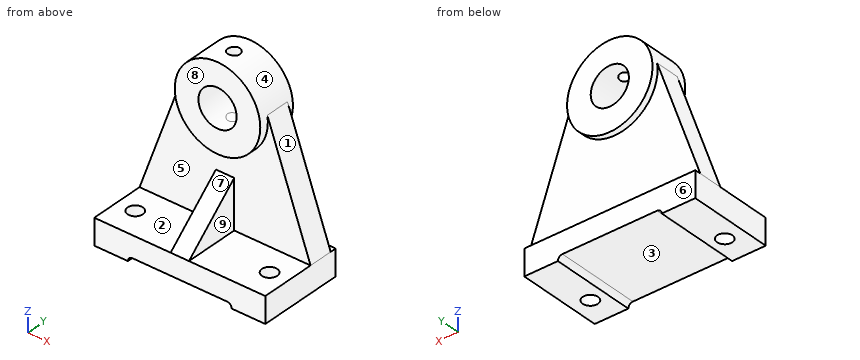
from build123d import *

# Parameters (mm, degrees)
F1_DEPTH  = 28
F3_DEPTH  = 28
F5_DEPTH  = 8
F7_DEPTH  = 4
F8_R      = 28
F9_DEPTH  = 28
F10_R     = 28
F11_DEPTH = 2
F12_R     = 12.5
F13_DEPTH = 26.001
F15_DEPTH = 112
F17_DEPTH = 50
F19_DEPTH = 50
F20_R     = 4
F21_DEPTH = 139
F22_R     = 4
F23_DEPTH = 91
F24_R     = 12.5
F25_DEPTH = 26.0010001
F26_R     = 5
F27_DEPTH = 120.0010001
F28_W     = 68
F28_H     = 3
F29_DEPTH = 28.0010001
F30_R     = 2.99999


# Not quite as in the source:
# - a fillet or chamfer is up to 0.001 mm smaller than in the source, because OpenCascade refuses the exact size


with BuildPart() as f1:
    # F0 (on Front) → F1 (new body, symmetric)
    with BuildSketch(Plane.XZ):
        Polygon((0, 17), (0, 0), (22, 0), (22, 3), (90, 3), (90, 0), (112, 0), (112, 17), align=None)
    extrude(amount=F1_DEPTH, both=True)

    # F2 (on Front) → F3 (join)
    with BuildSketch(Plane.XZ):
        with BuildLine():
            Line((28.3328655167, 96.304610259), (0, 17))
            Line((0, 17), (112, 17))
            Line((112, 17), (83.6671344833, 96.304610259))
            ThreePointArc((83.6671344833, 96.304610259), (56, 64), (28.3328655167, 96.304610259))
        make_face()
    extrude(amount=-F3_DEPTH)

    # F4 (on face) → F5 (cut)
    with BuildSketch(Plane.XZ):
        with BuildLine():
            ThreePointArc((83.6671344833, 96.304610259), (56, 64), (28.3328655167, 96.304610259))
            Line((28.3328655167, 96.304610259), (0, 17))
            Line((0, 17), (112, 17))
            Line((112, 17), (83.6671344833, 96.304610259))
        make_face()
    extrude(amount=-F5_DEPTH, mode=Mode.SUBTRACT)

    # F6 (on face) → F7 (cut)
    with BuildSketch(Plane(origin=(0, 28, 0), x_dir=(-1, 0, 0), z_dir=(0, 1, 0))):
        with BuildLine():
            Line((-83.6671344833, 96.304610259), (-112, 17))
            Line((-112, 17), (0, 17))
            Line((0, 17), (-28.3328655167, 96.304610259))
            ThreePointArc((-28.3328655167, 96.304610259), (-56, 64), (-83.6671344833, 96.304610259))
        make_face()
    extrude(amount=-F7_DEPTH, mode=Mode.SUBTRACT)

    # F8 (on Front) → F9 (join)
    with BuildSketch(Plane.XZ):
        with Locations((56, 92)):
            Circle(F8_R)
    extrude(amount=-F9_DEPTH)

    # F10 (on face) → F11 (cut)
    with BuildSketch(Plane.XZ):
        with Locations((56, 92)):
            Circle(F10_R)
    extrude(amount=-F11_DEPTH, mode=Mode.SUBTRACT)

    # F12 (on face) → F13 (cut, through all)
    with BuildSketch(Plane.XZ.offset(-2)):
        with Locations((56, 92)):
            Circle(F12_R)
    extrude(amount=-F13_DEPTH, mode=Mode.SUBTRACT)

    # F14 (on Right) → F15 (join)
    with BuildSketch(Plane.YZ):
        Polygon((8, 49), (-28, 17), (8, 17), align=None)
    extrude(amount=F15_DEPTH)

    # F16 (on face) → F17 (cut)
    with BuildSketch(Plane.YZ.offset(112)):
        Polygon((8, 49), (-28, 17), (8, 17), align=None)
    extrude(amount=-F17_DEPTH, mode=Mode.SUBTRACT)

    # F18 (on face) → F19 (cut)
    with BuildSketch(Plane(origin=(0, 0, 0), x_dir=(0, -1, 0), z_dir=(-1, 0, 0))):
        Polygon((-8, 49), (-8, 17), (28, 17), align=None)
    extrude(amount=-F19_DEPTH, mode=Mode.SUBTRACT)

    # F20 (on Top) → F21 (cut)
    with BuildSketch(Plane.XY):
        with Locations((56, 15)):
            Circle(F20_R)
    extrude(amount=F21_DEPTH, mode=Mode.SUBTRACT)

    # F22 (on Top) → F23 (join)
    with BuildSketch(Plane.XY):
        with Locations((56, 15)):
            Circle(F22_R)
    extrude(amount=F23_DEPTH)

    # F24 (on face) → F25 (cut, through all)
    with BuildSketch(Plane.XZ.offset(-2)):
        with Locations((56, 92)):
            Circle(F24_R)
    extrude(amount=-F25_DEPTH, mode=Mode.SUBTRACT)

    # F26 (on Top) → F27 (cut, through all)
    with BuildSketch(Plane.XY):
        with Locations((12, -10)):
            Circle(F26_R)
        with Locations((100, -10)):
            Circle(F26_R)
    extrude(amount=F27_DEPTH, mode=Mode.SUBTRACT)

    # F28 (on Front) → F29 (cut, through all)
    with BuildSketch(Plane.XZ):
        with Locations((56, 1.5)):
            Rectangle(F28_W, F28_H)
    extrude(amount=-F29_DEPTH, mode=Mode.SUBTRACT)

    # F30 (radius 3 in the source; OpenCascade refuses exactly that, so slightly less here)
    f30_edges = [f1.edges().sort_by_distance(p)[0] for p in [
        (90, 0, 3),
        (22, 0, 3),
    ]]
    fillet(f30_edges, radius=F30_R)


solid = f1.part
Design review of the part built by this model. Coordinates are the model's own, in mm. Face numbers are marked on the shaded views. A direction names the side the tool comes from. Coordinates: 2 decimals unless noted, no trailing zeros. Loops run counter-clockwise (first coordinate to the right, second up) from the corner with the lowest first, then second, coordinate; pieces in that order, holes last.
Item 1: Add section B-B (y = -10). Give the number of separate pieces and of enclosed holes in the cut face, and give its area (3 significant figures).
Completed:
separate pieces: 3
enclosed holes: 0
area: 1,560 mm2
Item 2: Add section C-C (z = 14). Write out the cut boundary in (x, y).
Completed:
outline: (0, -28) - (112, -28) - (112, 28) - (0, 28) - close; hole circle Ø10 at (12, -10); hole circle Ø10 at (100, -10)
Item 3: Draft analysis for pull direction X (two halves, no side actions). For the marked faces 1, 2, 3 and 4, state which applies: pulls with the +X half, pulls with the -X half, needs draft (parallel to the pull), parting line crosses it, or undercut.
Completed:
face 1: pulls with the +X half
face 2: needs draft
face 3: undercut
face 4: parting line crosses it
Item 4: Clearance check with flat-ended pins moving along their axes: pin 1 (12 mm diameter, centred on x = 56, y = -19, fed in from +Z); pin 2 (9 mm diameter, centred on x = 56, y = 15, fed in from +Z); pin 3 (1.2 mm diameter, centred on x = 66.5, y = 25.5, fed in from +Z); pin 4 (8 mm diameter, centred on x = 76.5, y = 0, fed in from +Z). State where each tip first meets the part, or that it passes through.
Completed:
pin 1: stops at z = 30.33
pin 2: stops at z = 120
pin 3: stops at z = 118.19
pin 4: stops at z = 114.22
Item 5: Add section A-A (x = 56). Write out the cut boundary in (y, z).
Completed:
outline: (-28, 3) - (28, 3) - (28, 17) - (24, 17) - (24, 64) - (28, 64) - (28, 79.5) - (2, 79.5) - (2, 64) - (8, 64) - (8, 49) - (-28, 17) - close; (2, 104.5) - (11, 104.5) - (11, 120) - (2, 120) - close; (19, 104.5) - (28, 104.5) - (28, 120) - (19, 120) - close
Item 6: For the marked faces 5, 6, 7, 8 and 9, list the 3-axis set-ups (+Z, -Z, +X, -X, +Y, -Y) from which the entire face can be reached by the end or side of a thin tool; tool diameter is ignored.
Completed:
face 5: -Y
face 6: +Z, -Z, +X, -X, +Y
face 7: +X, -X, -Y
face 8: +Z, +X, -X, -Y
face 9: +X, -Y
Item 7: Add section D-D (x = 14.5). Write out the cut boundary in (y, z).
Completed:
outline: (-28, 0) - (-14.33, 0) - (-14.33, 17) - (-28, 17) - close; (-5.67, 0) - (28, 0) - (28, 17) - (24, 17) - (24, 57.59) - (8, 57.59) - (8, 17) - (-5.67, 17) - close
Item 8: Wall thickness on L1, parallel to X at y = -10, z = 10; L2, parallel to Y at x = 12, z = 6; L3, parallel to Z at x = 56, y = 9.25: over which ranges is each line inside the solid? List them lowest first.
Completed:
L1: x = 0 to 7, 17 to 95, 105 to 112
L2: y = -28 to -15, -5 to 28
L3: z = 3 to 79.5, 104.5 to 120
